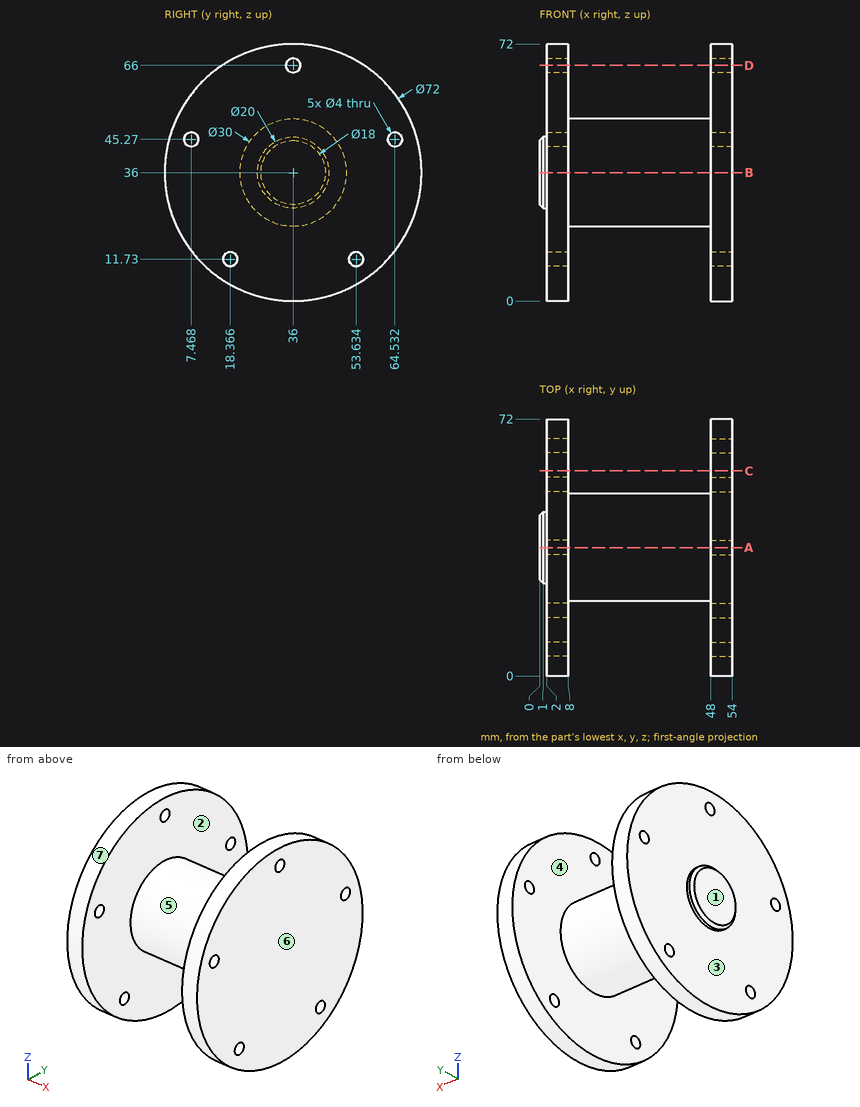
Check sheet for the drawn part. Datum: minimum x, y, z corner. Units: mm. A direction names the side the tool comes from. Give positions to 0.01 mm unless a question says otherwise; leave off trailing zeros. Write each loop counter-clockwise with the first axis right and the second up, starting at its lowest first coordinate (ties: lowest second). Pieces come first, ordered by that corner, then holes. Notation, with made-up numbers: M 42.5,-17.5 L 77.5,-17.5 A6 ccw 77.5,-7.5 Z; hole C 2.5,28.5 d1. An arc over 180 degrees is marked long. One line per question, with ' | ' between items.
1) Section check D-D on z = 66. Enter the section's corners in (x, y).
Result:
outline: M 2,16.1 L 8,16.1 L 8,34 L 2,34 Z; M 2,38 L 8,38 L 8,55.9 L 2,55.9 Z; M 48,16.1 L 54,16.1 L 54,34 L 48,34 Z; M 48,38 L 54,38 L 54,55.9 L 48,55.9 Z
2) Section check A-A on y = 36. Enter the section's corners in (x, z).
Result:
outline: M 0,27 L 1,26 L 2,26 L 2,0 L 8,0 L 8,21 L 48,21 L 48,0 L 54,0 L 54,64 L 48,64 L 48,51 L 8,51 L 8,64 L 2,64 L 2,46 L 1,46 L 0,45 Z; M 2,68 L 8,68 L 8,72 L 2,72 Z; M 48,68 L 54,68 L 54,72 L 48,72 Z
3) Set-up check for the marked faces 1, 2 and 3: record each of +Z, -Z, +X, -X, +Y, -Y from which the full face is reachable in a straight line by a thin tool's end or side.
Result:
face 1: +Z, -Z, -X, +Y, -Y | face 2: none | face 3: -X
4) Thickness scan on line 1 along X through (y, z) = (47, 59); line 2 along Z through (x, y) = (9, 35.5); line 3 along Y through (x, z) = (5, 66.5) (1 decimal). Record the ranges inside material, lowest first. Write a range as [from, to].
Result:
line 1: x = [2, 8], [48, 54] | line 2: z = [21.01, 50.99] | line 3: y = [16.9, 34.1], [37.9, 55.1]
5) Section check C-C on y = 57.5. Enter the section's corners in (x, z) (1 decimal).
Result:
outline: M 2,7.1 L 8,7.1 L 8,64.9 L 2,64.9 Z; M 48,7.1 L 54,7.1 L 54,64.9 L 48,64.9 Z
6) Gauge pin test, flat ends, axial feed: pin 1 Ø5 at (y, z) = (18.37, 11.73) entering from -X; pin 2 Ø1 at (x, y) = (48, 13) entering from +Z; pin 3 Ø6 at (x, y) = (22.5, 36) entering from +Z. Record the tip position at first contact, or that the pin passes through.
Result:
pin 1: stops at x = 2 | pin 2: stops at z = 64.1 | pin 3: stops at z = 51
7) Mould release check, pull along X, two halves, no side actions. Record for the marked faces 4, 5, 6 and 7: released by +X, released by -X, zero draft, split by the parting line, or undercut.
Result:
face 4: undercut | face 5: undercut | face 6: released by +X | face 7: zero draft
8) Section check B-B on z = 36. Enter the section's corners in (x, y).
Result:
outline: M 0,27 L 1,26 L 2,26 L 2,0 L 8,0 L 8,21 L 48,21 L 48,0 L 54,0 L 54,72 L 48,72 L 48,51 L 8,51 L 8,72 L 2,72 L 2,46 L 1,46 L 0,45 Z
